from build123d import *

# Parameters (mm, degrees)
SKETCH1_R                      = 61.976
BOSS_EXTRUDE1_DEPTH            = 6.35
F_1_1_DIAMETER_HOLE1_D         = 25.4
F_9_16_0_5625_DIAMETER_HOLE1_D = 14.2875


with BuildPart() as part:
    # Sketch1 → Boss-Extrude1 (new body)
    with BuildSketch(Plane.XY):
        Circle(SKETCH1_R)
    extrude(amount=BOSS_EXTRUDE1_DEPTH)

    # 1 (1) Diameter Hole1 (through all)
    with Locations(Plane.XY.offset(6.35)):
        with Locations((0, 0)):
            Hole(F_1_1_DIAMETER_HOLE1_D / 2)

    # 9/16 (0.5625) Diameter Hole1 (through all)
    with Locations(Plane.XY.offset(6.35)):
        with Locations((-43.994090512, -25.4), (43.994090512, -25.4), (0, 50.8)):
            Hole(F_9_16_0_5625_DIAMETER_HOLE1_D / 2)


solid = part.part
Geometry: final body of the model. Coordinates: model frame, mm. Round coordinates to 2 decimals unless told otherwise and drop trailing zeros. Loops run counter-clockwise (first coordinate to the right, second up) from the corner with the lowest first, then second, coordinate; pieces in that order, holes last. Notation, with made-up numbers: (-25, -13) - (25, -13) arc R15 ccw to (25, -5) - close; hole circle Ø2 at (55.5, 9.5). An arc over 180 degrees is marked (long way). Write each question's results on one line, items separated by ' | '. Start each with the question number.
1) Cut plane B-B on y = 0. Return loops of the section in (x, z).
2) Line query: probe 1 along Y at (x, z) = (0, 2); probe 2 along X at (y, z) = (-30.5, 5.75); probe 3 along X at (y, z) = (-27, 4.25). Output: solid intervals per line, ascending. Write a range as [from, to].
3) Cut plane A-A on x = 0. Return loops of the section in (y, z).
4) Mould query, pull axis Y, two halves, no side actions, for faces 1 (the face through (-1, -13, 6.35)), 2 (the face through (44.924, -18.317, 3.131)), 3 (the face through (33.318, 52.258, 3.131)). Classes: released by +Y, released by -Y, zero draft, split by the parting line, or undercut.
5) Cut plane D-D on z = 5.25. Return loops of the section in (x, y), then the cut area to 3 significant figures.
6) Cut plane C-C on y = -25.4. Return loops of the section in (x, z), then the cut area to 3 significant figures.
7) First-contact query: P1, Ø1.5, axis at y = -9.5, z = 1.5, coming from the +X side; P2, Ø11.5, axis at x = 0, y = 50.8, coming from the -Z side; P3, Ø2, axis at y = 4, z = 2.5, coming from the -X side. Flat tips, straight axial feed; report the tip coordinate or a pass-through.
Verdict:
1) outline: (-61.98, 0) - (-12.7, 0) - (-12.7, 6.35) - (-61.98, 6.35) - close; (12.7, 0) - (61.98, 0) - (61.98, 6.35) - (12.7, 6.35) - close
2) probe 1: y = [-61.98, -12.7], [12.7, 43.66], [57.94, 61.98] | probe 2: x = [-53.95, -49], [-38.99, 38.99], [49, 53.95] | probe 3: x = [-55.79, -50.96], [-37.03, 37.03], [50.96, 55.79]
3) outline: (-61.98, 0) - (-12.7, 0) - (-12.7, 6.35) - (-61.98, 6.35) - close; (12.7, 0) - (43.66, 0) - (43.66, 6.35) - (12.7, 6.35) - close; (57.94, 0) - (61.98, 0) - (61.98, 6.35) - (57.94, 6.35) - close
4) face 1: zero draft | face 2: undercut | face 3: split by the parting line
5) outline: circle Ø123.95 at (0, 0); hole circle Ø14.29 at (-43.99, -25.4); hole circle Ø25.4 at (0, 0); hole circle Ø14.29 at (0, 50.8); hole circle Ø14.29 at (43.99, -25.4) | area: 11,100 mm2
6) outline: (-56.53, 0) - (-51.14, 0) - (-51.14, 6.35) - (-56.53, 6.35) - close; (-36.85, 0) - (36.85, 0) - (36.85, 6.35) - (-36.85, 6.35) - close; (51.14, 0) - (56.53, 0) - (56.53, 6.35) - (51.14, 6.35) - close | area: 537 mm2
7) P1: stops at x = 61.36 | P2: passes through | P3: stops at x = -61.9
